```python
from build123d import *

# Parameters (mm, degrees)
SKETCH1_W                     = 90.17
SKETCH1_H                     = 55.88
BOSS_EXTRUDE1_DEPTH           = 27.94
SHELL1_T                      = -2.54
SKETCH2_R                     = 4.445
BOSS_EXTRUDE4_DEPTH           = 5.08
BOSS_EXTRUDE4_DRAFT           = 10
BOSS_EXTRUDE4_PROFILE_2_DEPTH = 5.08
BOSS_EXTRUDE4_PROFILE_2_DRAFT = 10
BOSS_EXTRUDE4_PROFILE_3_DEPTH = 5.08
BOSS_EXTRUDE4_PROFILE_3_DRAFT = 10
BOSS_EXTRUDE4_PROFILE_4_DEPTH = 5.08
BOSS_EXTRUDE4_PROFILE_4_DRAFT = 10
TAP_DRILL_FOR_4_40_TAP1_D     = 2.2606
TAP_DRILL_FOR_4_40_TAP1_DEPTH = 6.35
TAP_DRILL_FOR_4_40_TAP1_TIP   = 0.679152758
SKETCH6_R                     = 3.556
CUT_EXTRUDE1_DEPTH            = 2.54
CUT_EXTRUDE1_DRAFT            = 10
CUT_EXTRUDE1_PROFILE_2_DEPTH  = 2.54
CUT_EXTRUDE1_PROFILE_2_DRAFT  = 10
CUT_EXTRUDE1_PROFILE_3_DEPTH  = 2.54
CUT_EXTRUDE1_PROFILE_3_DRAFT  = 10
SKETCH6_R_2                   = 4.191
CUT_EXTRUDE1_PROFILE_4_DEPTH  = 2.54
CUT_EXTRUDE1_PROFILE_4_DRAFT  = 10
CUT_EXTRUDE1_PROFILE_5_DEPTH  = 2.54
CUT_EXTRUDE1_PROFILE_5_DRAFT  = 10
CUT_EXTRUDE2_REACH            = 100.448
SKETCH7_W                     = 9.017
SKETCH7_H                     = 11.176
SKETCH7_W_2                   = 7.874
SKETCH7_H_2                   = 3.81


with BuildPart() as part:
    # Sketch1 → Boss-Extrude1 (new body)
    with BuildSketch(Plane(origin=(0, 0, 0), x_dir=(1, 0, 0), z_dir=(0, 1, 0))):
        Rectangle(SKETCH1_W, SKETCH1_H)
    extrude(amount=BOSS_EXTRUDE1_DEPTH)

    # Shell1
    shell1_openings = [part.faces().sort_by_distance(p)[0] for p in [
        (0, 27.94, 0),
    ]]
    offset(amount=SHELL1_T, openings=shell1_openings, kind=Kind.INTERSECTION)


with BuildPart() as boss_extrude4_tool:
    # Sketch2 → Boss-Extrude4 (with draft: the straight prism first)
    with BuildSketch(Plane(origin=(0, 2.54, 0), x_dir=(1, 0, 0), z_dir=(0, 1, 0))):
        with Locations((37.465, 20.32)):
            Circle(SKETCH2_R)
    extrude(amount=BOSS_EXTRUDE4_DEPTH)
    # Boss-Extrude4: the draft: its side faces are tilted about the plane it starts from
    boss_extrude4_sides = [boss_extrude4_tool.faces().sort_by_distance(p)[0] for p in [
        (33.02, 5.08, -20.32),
    ]]
    draft(boss_extrude4_sides, Plane(origin=(0, 2.54, 0), x_dir=(1, 0, 0), z_dir=(0, 1, 0)), BOSS_EXTRUDE4_DRAFT)


with BuildPart() as part_1:
    add(part.part)

    # Boss-Extrude4: add boss_extrude4_tool
    add(boss_extrude4_tool.part)


with BuildPart() as boss_extrude4_profile_2_tool:
    # Sketch2 → Boss-Extrude4 profile 2 (with draft: the straight prism first)
    with BuildSketch(Plane(origin=(0, 2.54, 0), x_dir=(1, 0, 0), z_dir=(0, 1, 0))):
        with Locations((37.465, -20.32)):
            Circle(SKETCH2_R)
    extrude(amount=BOSS_EXTRUDE4_PROFILE_2_DEPTH)
    # Boss-Extrude4 profile 2: the draft: its side faces are tilted about the plane it starts from
    boss_extrude4_profile_2_sides = [boss_extrude4_profile_2_tool.faces().sort_by_distance(p)[0] for p in [
        (33.02, 5.08, 20.32),
    ]]
    draft(boss_extrude4_profile_2_sides, Plane(origin=(0, 2.54, 0), x_dir=(1, 0, 0), z_dir=(0, 1, 0)), BOSS_EXTRUDE4_PROFILE_2_DRAFT)


with BuildPart() as part_2:
    add(part_1.part)

    # Boss-Extrude4 profile 2: add boss_extrude4_profile_2_tool
    add(boss_extrude4_profile_2_tool.part)


with BuildPart() as boss_extrude4_profile_3_tool:
    # Sketch2 → Boss-Extrude4 profile 3 (with draft: the straight prism first)
    with BuildSketch(Plane(origin=(0, 2.54, 0), x_dir=(1, 0, 0), z_dir=(0, 1, 0))):
        with Locations((-36.195, -20.32)):
            Circle(SKETCH2_R)
    extrude(amount=BOSS_EXTRUDE4_PROFILE_3_DEPTH)
    # Boss-Extrude4 profile 3: the draft: its side faces are tilted about the plane it starts from
    boss_extrude4_profile_3_sides = [boss_extrude4_profile_3_tool.faces().sort_by_distance(p)[0] for p in [
        (-40.64, 5.08, 20.32),
    ]]
    draft(boss_extrude4_profile_3_sides, Plane(origin=(0, 2.54, 0), x_dir=(1, 0, 0), z_dir=(0, 1, 0)), BOSS_EXTRUDE4_PROFILE_3_DRAFT)


with BuildPart() as part_3:
    add(part_2.part)

    # Boss-Extrude4 profile 3: add boss_extrude4_profile_3_tool
    add(boss_extrude4_profile_3_tool.part)


with BuildPart() as boss_extrude4_profile_4_tool:
    # Sketch2 → Boss-Extrude4 profile 4 (with draft: the straight prism first)
    with BuildSketch(Plane(origin=(0, 2.54, 0), x_dir=(1, 0, 0), z_dir=(0, 1, 0))):
        with Locations((-36.195, 20.32)):
            Circle(SKETCH2_R)
    extrude(amount=BOSS_EXTRUDE4_PROFILE_4_DEPTH)
    # Boss-Extrude4 profile 4: the draft: its side faces are tilted about the plane it starts from
    boss_extrude4_profile_4_sides = [boss_extrude4_profile_4_tool.faces().sort_by_distance(p)[0] for p in [
        (-40.64, 5.08, -20.32),
    ]]
    draft(boss_extrude4_profile_4_sides, Plane(origin=(0, 2.54, 0), x_dir=(1, 0, 0), z_dir=(0, 1, 0)), BOSS_EXTRUDE4_PROFILE_4_DRAFT)


with BuildPart() as part_4:
    add(part_3.part)

    # Boss-Extrude4 profile 4: add boss_extrude4_profile_4_tool
    add(boss_extrude4_profile_4_tool.part)

    # Tap Drill for #4-40 Tap1
    with Locations(Plane(origin=(0, 7.62, 0), x_dir=(1, 0, 0), z_dir=(0, 1, 0))):
        with Locations((-36.195, 20.32), (-36.195, -20.32), (37.465, -20.32), (37.465, 20.32)):
            Hole(TAP_DRILL_FOR_4_40_TAP1_D / 2, depth=TAP_DRILL_FOR_4_40_TAP1_DEPTH)
            with Locations((0, 0, -(TAP_DRILL_FOR_4_40_TAP1_DEPTH + TAP_DRILL_FOR_4_40_TAP1_TIP / 2))):  # 118° drill point
                Cone(0, TAP_DRILL_FOR_4_40_TAP1_D / 2, TAP_DRILL_FOR_4_40_TAP1_TIP, mode=Mode.SUBTRACT)


with BuildPart() as cut_extrude1_tool:
    # Sketch6 → Cut-Extrude1 (with draft: the straight prism first)
    with BuildSketch(Plane.XY.offset(27.94)):
        with Locations((24.765, 16.256)):
            Circle(SKETCH6_R)
    extrude(amount=-CUT_EXTRUDE1_DEPTH)
    # Cut-Extrude1: the draft: its side faces are tilted about the plane it starts from
    cut_extrude1_sides = [cut_extrude1_tool.faces().sort_by_distance(p)[0] for p in [
        (21.209, 16.256, 26.67),
    ]]
    draft(cut_extrude1_sides, Plane.XY.offset(27.94), CUT_EXTRUDE1_DRAFT)


with BuildPart() as part_5:
    add(part_4.part)

    # Cut-Extrude1: cut by cut_extrude1_tool
    add(cut_extrude1_tool.part, mode=Mode.SUBTRACT)


with BuildPart() as cut_extrude1_profile_2_tool:
    # Sketch6 → Cut-Extrude1 profile 2 (with draft: the straight prism first)
    with BuildSketch(Plane.XY.offset(27.94)):
        with Locations((12.065, 16.256)):
            Circle(SKETCH6_R)
    extrude(amount=-CUT_EXTRUDE1_PROFILE_2_DEPTH)
    # Cut-Extrude1 profile 2: the draft: its side faces are tilted about the plane it starts from
    cut_extrude1_profile_2_sides = [cut_extrude1_profile_2_tool.faces().sort_by_distance(p)[0] for p in [
        (8.509, 16.256, 26.67),
    ]]
    draft(cut_extrude1_profile_2_sides, Plane.XY.offset(27.94), CUT_EXTRUDE1_PROFILE_2_DRAFT)


with BuildPart() as part_6:
    add(part_5.part)

    # Cut-Extrude1 profile 2: cut by cut_extrude1_profile_2_tool
    add(cut_extrude1_profile_2_tool.part, mode=Mode.SUBTRACT)


with BuildPart() as cut_extrude1_profile_3_tool:
    # Sketch6 → Cut-Extrude1 profile 3 (with draft: the straight prism first)
    with BuildSketch(Plane.XY.offset(27.94)):
        with Locations((-13.335, 16.256)):
            Circle(SKETCH6_R)
    extrude(amount=-CUT_EXTRUDE1_PROFILE_3_DEPTH)
    # Cut-Extrude1 profile 3: the draft: its side faces are tilted about the plane it starts from
    cut_extrude1_profile_3_sides = [cut_extrude1_profile_3_tool.faces().sort_by_distance(p)[0] for p in [
        (-16.891, 16.256, 26.67),
    ]]
    draft(cut_extrude1_profile_3_sides, Plane.XY.offset(27.94), CUT_EXTRUDE1_PROFILE_3_DRAFT)


with BuildPart() as part_7:
    add(part_6.part)

    # Cut-Extrude1 profile 3: cut by cut_extrude1_profile_3_tool
    add(cut_extrude1_profile_3_tool.part, mode=Mode.SUBTRACT)


with BuildPart() as cut_extrude1_profile_4_tool:
    # Sketch6 → Cut-Extrude1 profile 4 (with draft: the straight prism first)
    with BuildSketch(Plane.XY.offset(27.94)):
        with Locations((-0.635, 16.891)):
            Circle(SKETCH6_R_2)
    extrude(amount=-CUT_EXTRUDE1_PROFILE_4_DEPTH)
    # Cut-Extrude1 profile 4: the draft: its side faces are tilted about the plane it starts from
    cut_extrude1_profile_4_sides = [cut_extrude1_profile_4_tool.faces().sort_by_distance(p)[0] for p in [
        (-4.826, 16.891, 26.67),
    ]]
    draft(cut_extrude1_profile_4_sides, Plane.XY.offset(27.94), CUT_EXTRUDE1_PROFILE_4_DRAFT)


with BuildPart() as part_8:
    add(part_7.part)

    # Cut-Extrude1 profile 4: cut by cut_extrude1_profile_4_tool
    add(cut_extrude1_profile_4_tool.part, mode=Mode.SUBTRACT)


with BuildPart() as cut_extrude1_profile_5_tool:
    # Sketch6 → Cut-Extrude1 profile 5 (with draft: the straight prism first)
    with BuildSketch(Plane.XY.offset(27.94)):
        with Locations((-26.035, 16.891)):
            Circle(SKETCH6_R_2)
    extrude(amount=-CUT_EXTRUDE1_PROFILE_5_DEPTH)
    # Cut-Extrude1 profile 5: the draft: its side faces are tilted about the plane it starts from
    cut_extrude1_profile_5_sides = [cut_extrude1_profile_5_tool.faces().sort_by_distance(p)[0] for p in [
        (-30.226, 16.891, 26.67),
    ]]
    draft(cut_extrude1_profile_5_sides, Plane.XY.offset(27.94), CUT_EXTRUDE1_PROFILE_5_DRAFT)


with BuildPart() as part_9:
    add(part_8.part)

    # Cut-Extrude1 profile 5: cut by cut_extrude1_profile_5_tool
    add(cut_extrude1_profile_5_tool.part, mode=Mode.SUBTRACT)

    # Sketch7 → Cut-Extrude2 (cut, up to next)
    with BuildSketch(Plane(origin=(45.085, 0, 0), x_dir=(0, 0, -1), z_dir=(1, 0, 0)), mode=Mode.PRIVATE) as cut_extrude2_sk1:
        with Locations((10.16, 14.8082)):
            Rectangle(SKETCH7_W, SKETCH7_H)
    cut_extrude2_tool1 = extrude(cut_extrude2_sk1.sketch, amount=-CUT_EXTRUDE2_REACH, mode=Mode.PRIVATE) & part_9.part
    # Sketch7 → Cut-Extrude2 (cut, up to next)
    with BuildSketch(Plane(origin=(45.085, 0, 0), x_dir=(0, 0, -1), z_dir=(1, 0, 0)), mode=Mode.PRIVATE) as cut_extrude2_sk2:
        with Locations((-5.08, 23.749)):
            Rectangle(SKETCH7_W_2, SKETCH7_H_2)
    cut_extrude2_tool2 = extrude(cut_extrude2_sk2.sketch, amount=-CUT_EXTRUDE2_REACH, mode=Mode.PRIVATE) & part_9.part
    add(cut_extrude2_tool1.solids().sort_by_distance((45.085, 14.8082, -10.16))[0], mode=Mode.SUBTRACT)
    add(cut_extrude2_tool2.solids().sort_by_distance((45.085, 23.749, 5.08))[0], mode=Mode.SUBTRACT)


solid = part_9.part
```
Geometry: final body of the model. Coordinates: model frame, mm. A direction names the side the tool comes from. Coordinates: 2 decimals unless noted, no trailing zeros. Write each loop counter-clockwise with the first axis right and the second up, starting at its lowest first coordinate (ties: lowest second). Pieces come first, ordered by that corner, then holes. Notation, with made-up numbers: M 8,31.5 L 23,31.5 A17 ccw 23,42.5 Z; hole C 55,-31 d7. An arc over 180 degrees is marked long. Use CSV: the item, a comma, the result in double quotes. Start each with the question number.
1. Mould query, pull axis X, two halves, no side actions, for faces 5 (the face through (-1, 15, -25.4)), 6 (the face through (37, 7.62, 19)), 7 (the face through (44, 24, 9.017)), 8 (the face through (-45.085, 14, 0)). Classes: pulls with the +X half, pulls with the -X half, needs draft (parallel to the pull), parting line crosses it, or undercut.
2. Ray query, probe 1 along Z at (x, y) = (38, 14.5); probe 2 along X at (y, z) = (4, -12) (3 decimals); probe 3 along X at (y, z) = (5, -20.32) (3 decimals). Return the intervals inside material, ascending.
3. Cut plane A-A on z = 11. Return the cut outline in (x, y) (3 decimals), plus the area to 3 significant figures.
4. Reachability of faces 1 (the face through (-1, 14, -27.94)), 2 (the face through (-30.3, 17.1, 27.5)), 3 (the face through (42.545, 15, 0)), 4 (the face through (44, 20.396, -10)) from +Z, -Z, +X, -X, +Y, -Y: full face, straight path, thin tool, end or side. Return the list, or none.
5. First-contact query: P1, Ø5, axis at x = 1.5, z = 10.5, coming from the +Y side; P2, Ø3.5, axis at x = 36.5, z = -21.5, coming from the +Y side. Flat tips, straight axial feed; report the tip coordinate or a pass-through.
Entries:
1,face 5,"undercut"
1,face 6,"undercut"
1,face 7,"needs draft"
1,face 8,"pulls with the -X half"
2,probe 1,"-27.94 to -25.4, 25.4 to 27.94"
2,probe 2,"-45.085 to -42.545, 42.545 to 45.085"
2,probe 3,"-45.085 to -42.545, -40.206 to -37.325, -35.065 to -32.184, 33.454 to 36.335, 38.595 to 41.476, 42.545 to 45.085"
3,outline,"M -45.085,0 L 45.085,0 L 45.085,27.94 L 42.545,27.94 L 42.545,2.54 L -42.545,2.54 L -42.545,27.94 L -45.085,27.94 Z"
3,area,"358 mm²"
4,face 1,"-Z, +X, -X, +Y, -Y"
4,face 2,"none"
4,face 3,"+Y"
4,face 4,"+X"
5,P1,"y = 2.54"
5,P2,"y = 7.62"
